```python
from build123d import *

# Parameters (mm, degrees)
F0_W           = 41.402
F0_H           = 12.7
F1_DEPTH       = 57.15
F3_D           = 13.335
F3_CBORE_D     = 28.575
F3_CBORE_DEPTH = 1.6002
F2_W           = 34.798
F2_H           = 19.05
F4_DEPTH       = 47.6504
F6_DEPTH       = 34.9504
F7_W           = 19.05
F7_H           = 47.6504
F8_DEPTH       = 28.702
F9_W           = 19.05
F9_H           = 26.924
F10_DEPTH      = 19.05
F11_R          = 6.35
F14_D          = 6.35
F15_D          = 7.112


with BuildPart() as f1:
    # F0 (on Front) → F1 (new body)
    with BuildSketch(Plane.XZ):
        with Locations((20.701, 6.35)):
            Rectangle(F0_W, F0_H)
        Polygon((0, -3.175), (0, 0), (0, 12.7), (-12.7, 12.7), (-12.7, -3.175), align=None)
    extrude(amount=-F1_DEPTH)

    # F3 (through all)
    with Locations(Plane.XY.offset(12.7)):
        with Locations((19.05, 28.575)):
            CounterBoreHole(F3_D / 2, F3_CBORE_D / 2, F3_CBORE_DEPTH)

    # F2 (on face) → F4 (join)
    with BuildSketch(Plane.XY.offset(12.7)):
        with Locations((-30.099, 28.575)):
            Rectangle(F2_W, F2_H)
        Polygon((-3.048, 19.05), (-3.048, 28.575), (-3.048, 38.1), (-12.7, 38.1), (-12.7, 19.05), align=None)
    extrude(amount=F4_DEPTH)

    # F5 (on face) → F6 (cut)
    with BuildSketch(Plane.XZ.offset(-19.05)):
        Polygon((-3.048, 60.3504), (-47.498, 60.3504), (-3.048, 12.7), align=None)
    extrude(amount=-F6_DEPTH, mode=Mode.SUBTRACT)

    # F7 (on face) → F8 (join)
    with BuildSketch(Plane(origin=(-47.498, 0, 0), x_dir=(0, -1, 0), z_dir=(-1, 0, 0))):
        with Locations((-28.575, 36.5252)):
            Rectangle(F7_W, F7_H)
    extrude(amount=F8_DEPTH)

    # F9 (on face) → F10 (join)
    with BuildSketch(Plane.XZ.offset(-19.05)):
        with Locations((-66.675, 26.162)):
            Rectangle(F9_W, F9_H)
    extrude(amount=F10_DEPTH)

    # F11
    f11_edges = [f1.edges().sort_by_distance(p)[0] for p in [
        (-66.675, 0, 39.624),
    ]]
    fillet(f11_edges, radius=F11_R)

    # F14 (through all)
    with Locations(Plane.YZ.offset(-57.15)):
        with Locations((9.652, 28.702)):
            Hole(F14_D / 2)

    # F15 (through all)
    with Locations(Plane.XZ.offset(-19.05)):
        with Locations((-68.326, 50.6984)):
            Hole(F15_D / 2)


solid = f1.part
```
The model under review builds one solid part; all positions refer to its coordinate system, in mm. A direction names the side the tool comes from. Round coordinates to 2 decimals unless told otherwise and drop trailing zeros. Loops run counter-clockwise (first coordinate to the right, second up) from the corner with the lowest first, then second, coordinate; pieces in that order, holes last. Notation, with made-up numbers: (-21, 7) - (15, 7) arc R24 ccw to (15, 45) - close; hole circle Ø11 at (-29, 42.25). An arc over 180 degrees is marked (long way). Write each question's results on one line, items separated by ' | '. Start each with the question number.
Q1. Tool access review of faces 1 (the flat face through (20.4, 21.8, 0)), 2 (the flat face through (-67, 13, 39.624)), 3 (the cylindrical face through (26.731, 40.622, 11.911)): name each direction out of +Z, -Z, +X, -X, +Y, -Y from which nothing blocks a thin tool from reaching the whole face with its end or side.
Q2. Take a section at B-B on y = 15.5. Give the boundary of the cut face in (x, z) (3 decimals), plus the area to 3 significant figures.
Q3. Draft analysis for pull direction X (two halves, no side actions). For faces 4 (the flat face through (-25.584, 28.442, 36.859)), 5 (the flat face through (-6, 28, -3.175)), 6 (the flat face through (22, 22, 11.1)), state which applies: pulls with the +X half, pulls with the -X half, needs draft (parallel to the pull), parting line crosses it, or undercut.
Q4. Take a section at D-D on y = 5. Give the boundary of the cut face in (x, z) (3 decimals).
Q5. Insertion check: P1, Ø24, axis at x = -35, z = 34.5, coming from the +Y side; P2, Ø10, axis at x = 9.5, y = 25.5, coming from the -Z side; P3, Ø6, axis at x = -55.5, y = 23.5, coming from the -Z side. Each pin has a flat end and moves straight along its axis. Give the tip position at first contact, or say it passes through.
Q6. Take a section at A-A on x = 19.05. Give the boundary of the cut face in (y, z).
Q7. Wall thickness on line 1 along Z through (x, y) = (36, 21); line 2 along Z through (x, y) = (9, 37); line 3 along X through (y, z) = (17, 38): over which ranges is each line inside the solid? List them lowest first. Write a range as [from, to].
Data:
1) face 1: -Z, +X, +Y, -Y | face 2: +Z, +X, -X, -Y | face 3: +Z
2) outline: (-76.2, 12.7) - (-57.15, 12.7) - (-57.15, 39.624) - (-76.2, 39.624) - close; (-12.7, -3.175) - (0, -3.175) - (0, 0) - (41.402, 0) - (41.402, 12.7) - (24.81, 12.7) - (24.81, 11.1) - (13.29, 11.1) - (13.29, 12.7) - (-12.7, 12.7) - close | area: 1,220 mm²
3) face 4: pulls with the +X half | face 5: needs draft | face 6: undercut
4) outline: (-76.2, 12.7) - (-57.15, 12.7) - (-57.15, 39.479) - (-76.2, 39.479) - close; (-12.7, -3.175) - (0, -3.175) - (0, 0) - (41.402, 0) - (41.402, 12.7) - (-12.7, 12.7) - close
5) P1: stops at y = 38.1 | P2: stops at z = 0 | P3: stops at z = 12.7
6) outline: (0, 0) - (21.91, 0) - (21.91, 11.1) - (14.29, 11.1) - (14.29, 12.7) - (0, 12.7) - close; (35.24, 0) - (57.15, 0) - (57.15, 12.7) - (42.86, 12.7) - (42.86, 11.1) - (35.24, 11.1) - close
7) line 1: z = [0, 12.7] | line 2: z = [0, 11.1] | line 3: x = [-76.2, -57.15]
